```python
from build123d import *

# Parameters (mm, degrees)
CROQUIS1_W              = 110
CROQUIS1_H              = 90
SALIENTE_EXTRUIR1_DEPTH = 2
CROQUIS3_R              = 3
SALIENTE_EXTRUIR2_DEPTH = 5
CROQUIS4_R              = 1.5
CORTAR_EXTRUIR1_DEPTH   = 4
CROQUIS5_W              = 3
CROQUIS5_H              = 27
SALIENTE_EXTRUIR3_DEPTH = 19
CROQUIS6_W              = 3
CROQUIS6_H              = 36
CROQUIS6_H_2            = 13
CROQUIS6_H_3            = 10
SALIENTE_EXTRUIR4_DEPTH = 6
CROQUIS7_W              = 106
CROQUIS7_H              = 86
CROQUIS7_W_2            = 104
CROQUIS7_H_2            = 84
CORTAR_EXTRUIR2_DEPTH   = 5
CORTAR_EXTRUIR3_DEPTH   = 18
CROQUIS9_R              = 1.6
CORTAR_EXTRUIR4_DEPTH   = 12
CORTAR_EXTRUIR5_DEPTH   = 18
CROQUIS14_R             = 1.6
CORTAR_EXTRUIR6_DEPTH   = 10


with BuildPart() as part:
    # Croquis1 → Saliente-Extruir1 (new body)
    with BuildSketch(Plane(origin=(0, 0, 0), x_dir=(1, 0, 0), z_dir=(0, 1, 0))):
        Rectangle(CROQUIS1_W, CROQUIS1_H)
    extrude(amount=SALIENTE_EXTRUIR1_DEPTH)

    # Croquis3 → Saliente-Extruir2 (add)
    with BuildSketch(Plane(origin=(0, 2, 0), x_dir=(1, 0, 0), z_dir=(0, 1, 0))):
        with Locations(Location((-47.19, -37.19, 0), (0, 0, 90))):
            Circle(CROQUIS3_R)
        with Locations(Location((-47.19, 37.19, 0), (0, 0, 90))):
            Circle(CROQUIS3_R)
        with Locations(Location((35.36, -37.19, 0), (0, 0, 90))):
            Circle(CROQUIS3_R)
        with Locations(Location((35.36, 37.19, 0), (0, 0, 90))):
            Circle(CROQUIS3_R)
    extrude(amount=SALIENTE_EXTRUIR2_DEPTH)

    # Croquis4 → Cortar-Extruir1 (cut)
    with BuildSketch(Plane(origin=(0, 7, 0), x_dir=(1, 0, 0), z_dir=(0, 1, 0))):
        with Locations(Location((-47.19, -37.19, 0), (0, 0, 270))):
            Circle(CROQUIS4_R)
        with Locations(Location((35.36, -37.19, 0), (0, 0, 270))):
            Circle(CROQUIS4_R)
        with Locations(Location((35.36, 37.19, 0), (0, 0, 270))):
            Circle(CROQUIS4_R)
        with Locations(Location((-47.19, 37.19, 0), (0, 0, 270))):
            Circle(CROQUIS4_R)
    extrude(amount=-CORTAR_EXTRUIR1_DEPTH, mode=Mode.SUBTRACT)

    # Croquis5 → Saliente-Extruir3 (add)
    with BuildSketch(Plane(origin=(0, 2, 0), x_dir=(1, 0, 0), z_dir=(0, 1, 0))):
        Polygon((52, -37), (55, -37), (55, -45), (-55, -45), (-55, -17), (-52, -17), (-52, -42), (52, -42), align=None)
        Polygon((-55, 45), (55, 45), (55, 13), (52, 13), (52, 42), (-52, 42), (-52, 19), (-55, 19), align=None)
        with Locations((53.5, -13.5)):
            Rectangle(CROQUIS5_W, CROQUIS5_H)
    extrude(amount=SALIENTE_EXTRUIR3_DEPTH)

    # Croquis6 → Saliente-Extruir4 (add)
    with BuildSketch(Plane(origin=(0, 2, 0), x_dir=(1, 0, 0), z_dir=(0, 1, 0))):
        with Locations((-53.5, 1)):
            Rectangle(CROQUIS6_W, CROQUIS6_H)
        with Locations((53.5, 6.5)):
            Rectangle(CROQUIS6_W, CROQUIS6_H_2)
        with Locations((53.5, -32)):
            Rectangle(CROQUIS6_W, CROQUIS6_H_3)
    extrude(amount=SALIENTE_EXTRUIR4_DEPTH)

    # Croquis7 → Cortar-Extruir2 (cut)
    with BuildSketch(Plane(origin=(0, 21, 0), x_dir=(1, 0, 0), z_dir=(0, 1, 0))):
        Rectangle(CROQUIS7_W, CROQUIS7_H)
        Rectangle(CROQUIS7_W_2, CROQUIS7_H_2, mode=Mode.SUBTRACT)
    extrude(amount=-CORTAR_EXTRUIR2_DEPTH, mode=Mode.SUBTRACT)

    # Croquis8 → Cortar-Extruir3 (cut)
    with BuildSketch(Plane(origin=(0, 21, 0), x_dir=(1, 0, 0), z_dir=(0, 1, 0))):
        Polygon((55, -8.5), (54, -7.5), (54, -10.5), (55, -9.5), align=None)
        Polygon((55, 22.5), (55, 21.5), (54, 20.5), (54, 23.5), align=None)
    extrude(amount=-CORTAR_EXTRUIR3_DEPTH, mode=Mode.SUBTRACT)

    # Croquis9 → Cortar-Extruir4 (cut)
    with BuildSketch(Plane(origin=(55, 0, 0), x_dir=(0, 0, -1), z_dir=(1, 0, 0))):
        with Locations((-4.25, 13)):
            Circle(CROQUIS9_R)
        with Locations((17.25, 13)):
            Circle(CROQUIS9_R)
    extrude(amount=-CORTAR_EXTRUIR4_DEPTH, mode=Mode.SUBTRACT)

    # Croquis11 → Cortar-Extruir5 (cut)
    with BuildSketch(Plane(origin=(0, 21, 0), x_dir=(1, 0, 0), z_dir=(0, 1, 0))):
        Polygon((-55, -22.5), (-54, -21.5), (-54, -24.5), (-55, -23.5), align=None)
        Polygon((-55, 25.5), (-55, 24.5), (-54, 23.5), (-54, 26.5), align=None)
    extrude(amount=-CORTAR_EXTRUIR5_DEPTH, mode=Mode.SUBTRACT)

    # Croquis14 → Cortar-Extruir6 (cut)
    with BuildSketch(Plane.ZY.offset(55)):
        with Locations((-33, 13)):
            Circle(CROQUIS14_R)
        with Locations((31, 13)):
            Circle(CROQUIS14_R)
    extrude(amount=-CORTAR_EXTRUIR6_DEPTH, mode=Mode.SUBTRACT)


solid = part.part
```
Work out the finished part from the listing and answer in its coordinate system (mm). A direction names the side the tool comes from. Give positions to 0.01 mm unless a question says otherwise; leave off trailing zeros. Loops run counter-clockwise (first coordinate to the right, second up) from the corner with the lowest first, then second, coordinate; pieces in that order, holes last. Notation, with made-up numbers: M 77,52.5 L 89,52.5 A11 ccw 89,72.5 Z; hole C 2.5,-23.75 d9. An arc over 180 degrees is marked long. One line per item, written item: value. Start each with the question number.
1. Find section A-A (z = -33). Give the vertices of the cut face in (x, y), and give its area (3 significant figures).
2. Each of these flat-tipped pins is pushed along its axis until it touches: P1, Ø0.9, axis at x = 35.5, z = 38, coming from the +Y side; P2, Ø1.8, axis at x = -47, z = 38, coming from the +Y side; P3, Ø5, axis at x = -39, z = 10.5, coming from the +Y side. Where does it stop, or does it pass through?
3. Find section C-C (z = -6). Give the vertices of the cut face in (x, y), and give its area (3 significant figures).
4. Find the intervals of material crossed by probe 1 along X at (y, z) = (5.1, -37.19); probe 2 along Z at (x, y) = (28, 5); probe 3 along X at (y, z) = (6.25, 31), in increasing order.
5. Determine the mould class of faces 1 (the face through (1, 10, 45)), 2 (the face through (55, 6, -1)), 3 (the face through (-47, 3, -37)), 4 (the face through (36, 7, 39)) for opening direction X: released by +X, released by -X, zero draft, split by the parting line, or undercut.
6. Find section B-B (x = 20). Give the vertices of the cut face in (y, z).
7. Find section D-D (y = 13). State how many separate pieces and enclosed holes the cut face has, and give its area (3 significant figures).
8. Which of the six approach directions +Z, -Z, +X, -X, +Y, -Y give full straight-line access (tool end or side, diameter ignored) to faces 5 (the face through (38.29, 4.46, 37.84)), 6 (the face through (53, 14, 0)), 7 (the face through (-53, 14, -19)), 8 (the face through (-55, 6, 1))?
Reported:
1. outline: M -55,0 L 55,0 L 55,21 L 53,21 L 53,16 L 52,16 L 52,2 L -52,2 L -52,11.4 L -55,11.4 Z; M -55,14.6 L -52,14.6 L -52,16 L -53,16 L -53,21 L -55,21 Z
1. area: 314 mm²
2. P1: stops at y = 3
2. P2: stops at y = 7
2. P3: stops at y = 2
3. outline: M -55,0 L 55,0 L 55,8 L 52,8 L 52,2 L -52,2 L -52,8 L -55,8 Z
3. area: 256 mm²
4. probe 1: x = -55 to -52, -50.19 to -48.69, -45.69 to -44.19, 32.36 to 33.86, 36.86 to 38.36, 52 to 55
4. probe 2: z = -45 to -42, 42 to 45
4. probe 3: x = -55 to -52, 52 to 55
5. face 1: zero draft
5. face 2: released by +X
5. face 3: undercut
5. face 4: undercut
6. outline: M 0,-45 L 21,-45 L 21,-43 L 16,-43 L 16,-42 L 2,-42 L 2,42 L 16,42 L 16,43 L 21,43 L 21,45 L 0,45 Z
7. separate pieces: 7
7. enclosed holes: 0
7. area: 941 mm²
8. face 5: +Y
8. face 6: +X, -X, +Y
8. face 7: -X, +Y
8. face 8: +Z, -Z, -X, +Y, -Y
